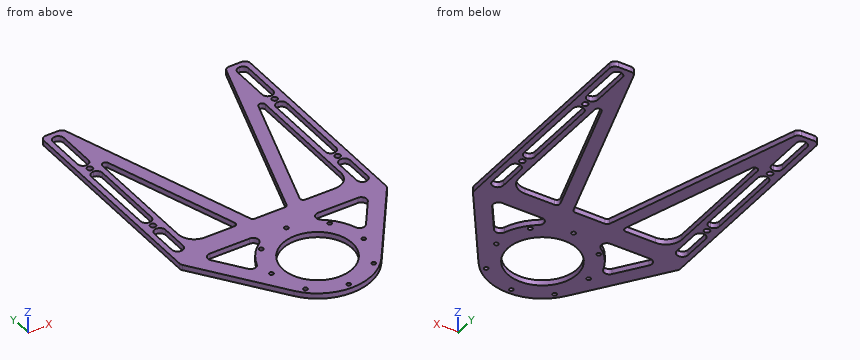
```python
from build123d import *

# Parameters (mm, degrees)
SKETCH_1_W          = 20
SKETCH_1_H          = 200
SKETCH_1_R          = 28.5
EXTRUDE_1_DEPTH     = 2.5
CUT_EXTRUDE_2_DEPTH = 10
EXTRUDE_2_DEPTH     = 5
SKETCH_4_R          = 2.6
CUT_EXTRUDE_3_DEPTH = 10
SKETCH_5_W          = 150
SKETCH_5_H          = 20
EXTRUDE_3_DEPTH     = 5
FILLET_1_R          = 15
CUT_EXTRUDE_START   = -10
SKETCH_6_W          = 10
SKETCH_6_H          = 45
SKETCH_6_H_2        = 80
SKETCH_6_R          = 32
SKETCH_6_R_2        = 28.5
CUT_EXTRUDE_4_DEPTH = 10
CUT_EXTRUDE_5_DEPTH = 10
SKETCH_8_R          = 1.9
CUT_EXTRUDE_6_DEPTH = 10
EXTRUDE_4_DEPTH     = 5
FILLET_3_R          = 3
CUT_EXTRUDE_9_DEPTH = 14
FILLET_4_R          = 5
FILLET_5_R          = 5


with BuildPart() as part:
    # 草图1 → 凸台-拉伸1 (new, symmetric)
    # profile 1 of 3: a face of its own
    with BuildSketch(Plane.XY):
        with Locations((-85, 100)):
            Rectangle(SKETCH_1_W, SKETCH_1_H)
    # profile 2 of 3: a face of its own
    with BuildSketch(Plane.XY):
        Polygon((-75, 0), (-95, 0), (-95, -83), (95, -83), (95, 0), (75, 0), align=None)
        with Locations((0, -48)):
            Circle(SKETCH_1_R, mode=Mode.SUBTRACT)
    # profile 3 of 3: a face of its own
    with BuildSketch(Plane.XY):
        with Locations((85, 100)):
            Rectangle(SKETCH_1_W, SKETCH_1_H)
    extrude(amount=EXTRUDE_1_DEPTH, both=True)

    # 草图2 → 切除-拉伸2 (cut)
    with BuildSketch(Plane.XY.offset(2.5)):
        with BuildLine():
            Line((-25.660561099, -72.531318841), (-95, 0))
            Line((-95, 0), (-95, -83))
            Line((-95, -83), (-5.937171044, -83))
            ThreePointArc((-5.937171044, -83), (-16.643391795, -79.356777729), (-25.660561099, -72.531318841))
        make_face()
        with BuildLine():
            Line((95, 0), (25.660561099, -72.531318841))
            ThreePointArc((25.660561099, -72.531318841), (16.643391795, -79.356777729), (5.937171044, -83))
            Line((5.937171044, -83), (95, -83))
            Line((95, -83), (95, 0))
        make_face()
    extrude(amount=-CUT_EXTRUDE_2_DEPTH, mode=Mode.SUBTRACT)

    # 草图3 → 凸台-拉伸2 (add)
    with BuildSketch(Plane.XY.offset(2.5)):
        with BuildLine():
            Line((-95, 0), (-40.308710858, -76.730781907))
            ThreePointArc((-40.308710858, -76.730781907), (0, -97.5), (40.308710858, -76.730781907))
            Line((40.308710858, -76.730781907), (95, 0))
            Line((95, 0), (25.660561099, -72.531318841))
            ThreePointArc((25.660561099, -72.531318841), (16.643391795, -79.356777729), (5.937171044, -83))
            Line((5.937171044, -83), (-5.937171044, -83))
            ThreePointArc((-5.937171044, -83), (-16.643391795, -79.356777729), (-25.660561099, -72.531318841))
            Line((-25.660561099, -72.531318841), (-95, 0))
        make_face()
        with BuildLine():
            ThreePointArc((12.093386622, 0), (0, 1.5), (-12.093386622, 0))
            Line((-12.093386622, 0), (12.093386622, 0))
        make_face()
    extrude(amount=-EXTRUDE_2_DEPTH)

    # 草图4 → 切除-拉伸3 (cut)
    with BuildSketch(Plane.XY.offset(2.5)):
        with Locations((85, 145)):
            Circle(SKETCH_4_R)
        with Locations((85, 55)):
            Circle(SKETCH_4_R)
    cut_extrude_3 = extrude(amount=-CUT_EXTRUDE_3_DEPTH, mode=Mode.SUBTRACT)

    # 镜向1: 切除-拉伸3 across plane
    add(cut_extrude_3.mirror(Plane(origin=(0, 0, 0), x_dir=(0, 0, 1), z_dir=(1, 0, 0))), mode=Mode.SUBTRACT)

    # 草图5 → 凸台-拉伸3 (add)
    with BuildSketch(Plane.XY.offset(2.5)):
        with Locations((0, 10)):
            Rectangle(SKETCH_5_W, SKETCH_5_H)
    extrude(amount=-EXTRUDE_3_DEPTH)

    # 圆角1
    fillet_1_edges = [part.edges().sort_by_distance(p)[0] for p in [
        (-75, 20, 0),
        (75, 20, 0),
    ]]
    fillet(fillet_1_edges, radius=FILLET_1_R)

    # 草图6 → 切除-拉伸4 (cut)
    # profile 1 of 5: a face of its own
    with BuildSketch(Plane.XY.offset(2.5).offset(CUT_EXTRUDE_START)):
        with Locations((-85, 172.5)):
            Rectangle(SKETCH_6_W, SKETCH_6_H)
    # profile 2 of 5: a face of its own
    with BuildSketch(Plane.XY.offset(2.5).offset(CUT_EXTRUDE_START)):
        with Locations((-85, 100)):
            Rectangle(SKETCH_6_W, SKETCH_6_H_2)
    # profile 3 of 5: a face of its own
    with BuildSketch(Plane.XY.offset(2.5).offset(CUT_EXTRUDE_START)):
        with Locations((85, 100)):
            Rectangle(SKETCH_6_W, SKETCH_6_H_2)
    # profile 4 of 5: a face of its own
    with BuildSketch(Plane.XY.offset(2.5).offset(CUT_EXTRUDE_START)):
        with Locations((85, 172.5)):
            Rectangle(SKETCH_6_W, SKETCH_6_H)
    # profile 5 of 5: a face of its own
    with BuildSketch(Plane.XY.offset(2.5).offset(CUT_EXTRUDE_START)):
        with Locations((0, -48)):
            Circle(SKETCH_6_R)
        with Locations((0, -48)):
            Circle(SKETCH_6_R_2, mode=Mode.SUBTRACT)
    extrude(amount=CUT_EXTRUDE_4_DEPTH, mode=Mode.SUBTRACT)

    # 草图7 → 切除-拉伸5 (cut)
    with BuildSketch(Plane.XY.offset(2.5)):
        with BuildLine():
            Line((-79.89229429, 45), (-79.89229429, 20))
            ThreePointArc((-79.89229429, 20), (-85, 14.89229429), (-90.10770571, 20))
            Line((-90.10770571, 20), (-90.10770571, 45))
            ThreePointArc((-90.10770571, 45), (-85, 50.10770571), (-79.89229429, 45))
        make_face()
        with BuildLine():
            Line((90.10770571, 45), (90.10770571, 20))
            ThreePointArc((90.10770571, 20), (85, 14.89229429), (79.89229429, 20))
            Line((79.89229429, 20), (79.89229429, 45))
            ThreePointArc((79.89229429, 45), (85, 50.10770571), (90.10770571, 45))
        make_face()
    extrude(amount=-CUT_EXTRUDE_5_DEPTH, mode=Mode.SUBTRACT)

    # 草图8 → 切除-拉伸6 (cut)
    with BuildSketch(Plane.XY.offset(2.5)):
        with Locations((0, -3.5)):
            Circle(SKETCH_8_R)
        with Locations((31.466251763, -16.533748237)):
            Circle(SKETCH_8_R)
        with Locations((31.466251763, -79.466251763)):
            Circle(SKETCH_8_R)
        with Locations((0, -92.5)):
            Circle(SKETCH_8_R)
        with Locations((-31.466251763, -79.466251763)):
            Circle(SKETCH_8_R)
        with Locations((-31.466251763, -16.533748237)):
            Circle(SKETCH_8_R)
        with Locations((-42.5, -48)):
            Circle(SKETCH_8_R)
        with Locations((42.5, -48)):
            Circle(SKETCH_8_R)
    extrude(amount=-CUT_EXTRUDE_6_DEPTH, mode=Mode.SUBTRACT)

    # 草图9 → 凸台-拉伸4 (add)
    with BuildSketch(Plane.XY.offset(2.5)):
        Polygon((-15.981567349, 20), (-75, 200), (-75, 161.484192434), (-28.61013732, 20), align=None)
    extrude_4 = extrude(amount=-EXTRUDE_4_DEPTH)

    # 镜向2: 凸台-拉伸4 across plane
    add(extrude_4.mirror(Plane(origin=(0, 0, 0), x_dir=(0, 0, 1), z_dir=(1, 0, 0))))

    # 圆角3
    fillet_3_edges = [part.edges().sort_by_distance(p)[0] for p in [
        (-75, 161.484192434, 0),
        (-15.981567349, 20, 0),
        (-28.61013732, 20, 0),
        (75, 161.484192434, 0),
        (28.61013732, 20, 0),
        (15.981567349, 20, 0),
    ]]
    fillet(fillet_3_edges, radius=FILLET_3_R)

    # 草图11 → 切除-拉伸9 (cut)
    with BuildSketch(Plane.XY.offset(2.5)):
        with BuildLine():
            Line((-77.807686347, 0), (-47.883202974, -41.983450078))
            ThreePointArc((-47.883202974, -41.983450078), (-33.761084244, -13.515377475), (-5, 0))
            Line((-5, 0), (-77.807686347, 0))
        make_face()
        with BuildLine():
            Line((77.807686347, 0), (5, 0))
            ThreePointArc((5, 0), (33.761084244, -13.515377475), (47.883202974, -41.983450078))
            Line((47.883202974, -41.983450078), (77.807686347, 0))
        make_face()
    extrude(amount=-CUT_EXTRUDE_9_DEPTH, mode=Mode.SUBTRACT)

    # 圆角4
    fillet_4_edges = [part.edges().sort_by_distance(p)[0] for p in [
        (-47.883202974, -41.983450078, 0),
        (-5, 0, 0),
        (-80, 60, 0),
        (-90, 60, 0),
        (-90, 140, 0),
        (-80, 140, 0),
        (80, 150, 0),
        (80, 195, 0),
        (90, 195, 0),
        (90, 150, 0),
        (-90, 195, 0),
        (-80, 195, 0),
        (-80, 150, 0),
        (-90, 150, 0),
        (90, 60, 0),
        (80, 60, 0),
        (80, 140, 0),
        (90, 140, 0),
        (5, 0, 0),
        (77.807686347, 0, 0),
        (47.883202974, -41.983450078, 0),
        (-77.807686347, 0, 0),
    ]]
    fillet(fillet_4_edges, radius=FILLET_4_R - 0.0001)  # a hair under: the kernel refuses the full size

    # 圆角5
    fillet_5_edges = [part.edges().sort_by_distance(p)[0] for p in [
        (-95, 200, 0),
        (-75, 200, 0),
        (75, 200, 0),
        (95, 200, 0),
        (-95, 0, 0),
        (95, 0, 0),
    ]]
    fillet(fillet_5_edges, radius=FILLET_5_R)


solid = part.part
```
Geometry: final body of the model. Coordinates: model frame, mm. Give positions to 0.01 mm unless a question says otherwise; leave off trailing zeros. Write each loop counter-clockwise with the first axis right and the second up, starting at its lowest first coordinate (ties: lowest second). Pieces come first, ordered by that corner, then holes.
1. Section query B-B, the plane y = -62. Return loops of the section in (x, z), then the cut area to 3 significant figures.
2. Section query A-A, the plane y = -22. Return loops of the section in (x, z).
3. Section query C-C, the plane y = 90.5. Return loops of the section in (x, z), then the cut area to 3 significant figures.
4. Pin query (flat end, axial travel): P1, Ø1.5, axis at y = -15.5, z = 0, coming from the +X side; P2, Ø1, axis at x = 40, y = 53, coming from the +Z side; P3, Ø1, axis at y = -11, z = -2, coming from the -X side; P4, Ø2, axis at y = -63.5, z = -1.5, coming from the -X side. Return the tip coordinate at first contact, or that it passes through.
5. Section query D-D, the plane z = -0.3. Count the separate pieces of the cut face and the enclosed holes in it, then the cut area to 3 significant figures.
6. Line query: probe 1 along X at (y, z) = (19, 0.85); probe 2 along Y at (x, z) = (0, 0.8); probe 3 along X at (y, z) = (106, -1.55). Output: solid intervals per line, ascending.
Computed:
1. outline: (-50.81, -2.5) - (-28.77, -2.5) - (-28.77, 2.5) - (-50.81, 2.5) - close; (28.77, -2.5) - (50.81, -2.5) - (50.81, 2.5) - (28.77, 2.5) - close
1. area: 220 mm2
2. outline: (-79.32, -2.5) - (-62.13, -2.5) - (-62.13, 2.5) - (-79.32, 2.5) - close; (-40.66, -2.5) - (-18.65, -2.5) - (-18.65, 2.5) - (-40.66, 2.5) - close; (18.65, -2.5) - (40.66, -2.5) - (40.66, 2.5) - (18.65, 2.5) - close; (62.13, -2.5) - (79.32, -2.5) - (79.32, 2.5) - (62.13, 2.5) - close
3. outline: (-95, -2.5) - (-90, -2.5) - (-90, 2.5) - (-95, 2.5) - close; (-80, -2.5) - (-75, -2.5) - (-75, 2.5) - (-80, 2.5) - close; (-51.73, -2.5) - (-39.1, -2.5) - (-39.1, 2.5) - (-51.73, 2.5) - close; (39.1, -2.5) - (51.73, -2.5) - (51.73, 2.5) - (39.1, 2.5) - close; (75, -2.5) - (80, -2.5) - (80, 2.5) - (75, 2.5) - close; (90, -2.5) - (95, -2.5) - (95, 2.5) - (90, 2.5) - close
3. area: 226 mm2
4. P1: stops at x = 84.49
4. P2: passes through
4. P3: stops at x = -87.52
4. P4: stops at x = -50.45
5. separate pieces: 1
5. enclosed holes: 23
5. area: 18,300 mm2
6. probe 1: x = -95 to -90.01, -79.99 to 79.99, 90.01 to 95
6. probe 2: y = -97.5 to -94.4, -90.6 to -80, -16 to -5.4, -1.6 to 20
6. probe 3: x = -95 to -90, -80 to -75, -56.81 to -44.18, 44.18 to 56.81, 75 to 80, 90 to 95
